Check sheet for the modelled part. Datum: model origin and axes. Units: mm. A direction names the side the tool comes from. Give positions to 0.01 mm unless a question says otherwise; leave off trailing zeros. Order: outer loops, then holes, each group sorted by start corner. A loop starts at its lowest first (then second) coordinate and runs counter-clockwise, first axis right, second up.
Item 1: Sectioned sample at B-B on x = -0.5. Record the boundary of the cut face in (y, z).
Item 2: Sectioned sample at A-A on z = 0. Record the boundary of the cut face in (x, y).
Item 3: Sectioned sample at D-D on y = 7.5. Record the boundary of the cut face in (x, z), and give its area (3 significant figures).
Item 4: Access from +Z, -Z, +X, -X, +Y, -Y to the whole of each face (thin tool, end or side, straight path). Record for faces 1 (the cylindrical face through (3, 31, 0)), 2 (the flat face through (0, 0, 0)).
Item 5: Gauge pin test, flat ends, axial feed: P1, Ø1, axis at x = -2.5, y = 13.5, coming from the -Z side; P2, Ø1, axis at y = 14.5, z = -2, coming from the +X side; P3, Ø3, axis at y = 5.5, z = 2.5, coming from the -X side. Record the tip position at first contact, or that the pin passes through.
Item 6: Material ranges on line 1 along Y through (x, z) = (2.5, 1.75); line 2 along X through (y, z) = (17, 0); line 3 along Z through (x, y) = (-1, 28), recorded low to high.
Item 7: Sectioned sample at C-C on y = 40. Record the boundary of the cut face in (x, z).
Autodesk Inventor part; units mm, degrees
ref_plane "YZ Plane" through (0, 0, 0) normal (1, 0, 0) x (0, 1, 0)
ref_plane "XZ Plane" through (0, 0, 0) normal (0, 1, 0) x (-1, 0, 0)
ref_plane "XY Plane" through (0, 0, 0) normal (0, 0, 1) x (1, 0, 0)
sketch "Sketch1" plane through (0, 0, 0) normal (0, 1, 0) x (-1, 0, 0)
  circle A0 centre (0, 0) radius 3
  dimension "d0" = 6
extrude "Extrusion1" add sketch "Sketch1" along normal blind 50
fillet "Fillet1" radius 3 1 edges at (3, 50, 0)
sketch "Sketch2" plane through (0, 0, 0) normal (0, -1, 0) x (1, 0, 0)
  circle A0 centre (0, 0) radius 3.25
  dimension "d4" = 6.5
extrude "Extrusion2" add sketch "Sketch2" against normal blind 15
properties part number "Temp Water Sensor"
Report:
1. outline: (0, -3.21) - (15, -3.21) - (15, -2.96) - (47, -2.96) arc R2.96 ccw to (47, 2.96) - (15, 2.96) - (15, 3.21) - (0, 3.21) - close
2. outline: (-3.25, 0) - (3.25, 0) - (3.25, 15) - (3, 15) - (3, 47) arc R3 ccw to (-3, 47) - (-3, 15) - (-3.25, 15) - close
3. outline: circle Ø6.5 at (0, 0)
3. area: 33.2 mm2
4. face 1: +Y
4. face 2: +Z, -Z, +X, -X, -Y
5. P1: stops at z = -2.56
5. P2: stops at x = 2.88
5. P3: stops at x = -3.09
6. line 1: y = 0 to 15
6. line 2: x = -3 to 3
6. line 3: z = -2.83 to 2.83
7. outline: circle Ø6 at (0, 0)
